from build123d import *

# Parameters (mm, degrees)
BOSS_EXTRUDE1_DEPTH      = 22
BOSS_EXTRUDE1_DEPTH_BACK = 54
SKETCH1_W                = 213
SKETCH1_H                = 136
SKETCH2_W                = 18
SKETCH2_H                = 18
CUT_EXTRUDE1_DEPTH       = 15
CUT_EXTRUDE2_DEPTH       = 12.84
CUT_EXTRUDE3_DEPTH       = 12.84
CUT_EXTRUDE4_DEPTH       = 181.981352631
SKETCH9_R                = 1.905
CUT_EXTRUDE8_DEPTH       = 5
SKETCH11_R               = 4.445
CUT_EXTRUDE10_DEPTH      = 137.921009741


with BuildPart() as part:
    # Sketch1 → Boss-Extrude1 (new, two sides: drawn at the far end of the back side and taken through both)
    with BuildSketch(Plane(origin=(0, 0, 0), x_dir=(1, 0, 0), z_dir=(0, 1, 0)).offset(-BOSS_EXTRUDE1_DEPTH_BACK)):
        Rectangle(SKETCH1_W, SKETCH1_H)
    extrude(amount=BOSS_EXTRUDE1_DEPTH + BOSS_EXTRUDE1_DEPTH_BACK)

    # Sketch2 → Cut-Extrude1 (cut)
    with BuildSketch(Plane(origin=(0, 22, 0), x_dir=(1, 0, 0), z_dir=(0, 1, 0))):
        with Locations((-85.5, 43)):
            Rectangle(SKETCH2_W, SKETCH2_H)
        with Locations((-85.5, -43)):
            Rectangle(SKETCH2_W, SKETCH2_H)
        with Locations((57.5, 43)):
            Rectangle(SKETCH2_W, SKETCH2_H)
        with Locations((57.5, -43)):
            Rectangle(SKETCH2_W, SKETCH2_H)
    extrude(amount=-CUT_EXTRUDE1_DEPTH, mode=Mode.SUBTRACT)

    # Sketch4 → Cut-Extrude2 (cut)
    with BuildSketch(Plane.ZY.offset(76.5)):
        Polygon((34, 7), (52, 7), (52, 11), (48.05, 11), (48.05, 24.194829177), (37.95, 24.194829177), (37.95, 11), (34, 11), align=None)
        Polygon((-34, 7), (-52, 7), (-52, 11), (-48.05, 11), (-48.05, 24.194829177), (-37.95, 24.194829177), (-37.95, 11), (-34, 11), align=None)
    extrude(amount=-CUT_EXTRUDE2_DEPTH, mode=Mode.SUBTRACT)

    # Sketch5 → Cut-Extrude3 (cut)
    with BuildSketch(Plane.ZY.offset(-66.5)):
        Polygon((34, 7), (52, 7), (52, 11), (48.05, 11), (48.05, 24.194829177), (37.95, 24.194829177), (37.95, 11), (34, 11), align=None)
        Polygon((-34, 7), (-52, 7), (-52, 11), (-48.05, 11), (-48.05, 24.194829177), (-37.95, 24.194829177), (-37.95, 11), (-34, 11), align=None)
    extrude(amount=-CUT_EXTRUDE3_DEPTH, mode=Mode.SUBTRACT)

    # Sketch7 → Cut-Extrude4 (cut, through all)
    with BuildSketch(Plane(origin=(0, 0, -68), x_dir=(-1, 0, 0), z_dir=(0, 0, -1))):
        Polygon((106.5, -54), (-106.5, 3.073177988), (-106.5, -54), align=None)
    extrude(amount=-CUT_EXTRUDE4_DEPTH, mode=Mode.SUBTRACT)

    # Sketch9 → Cut-Extrude8 (cut)
    with BuildSketch(Plane(origin=(6.365852752, -23.757685902, 0), x_dir=(0.9659258262890681, 0.2588190451025214, 0), z_dir=(0.2588190451025214, -0.9659258262890681, 0))):
        with Locations((-61.719828935, 0)):
            Circle(SKETCH9_R)
        with Locations((48.538997492, 0)):
            Circle(SKETCH9_R)
    extrude(amount=-CUT_EXTRUDE8_DEPTH, mode=Mode.SUBTRACT)

    # Sketch11 → Cut-Extrude10 (cut, through all)
    with BuildSketch(Plane(origin=(5.071757526, -18.928056771, 0), x_dir=(0.9659258262890681, 0.25881904510252135, 0), z_dir=(0.25881904510252135, -0.9659258262890681, 0))):
        with Locations((-61.719828935, 0)):
            Circle(SKETCH11_R)
        with Locations((48.538997492, 0)):
            Circle(SKETCH11_R)
    extrude(amount=-CUT_EXTRUDE10_DEPTH, mode=Mode.SUBTRACT)


solid = part.part
CAD build for the part. Positions are in the model's coordinates, mm. A direction names the side the tool comes from. Coordinates: 2 decimals unless noted, no trailing zeros. Order: outer loops, then holes, each group sorted by start corner. A loop starts at its lowest first (then second) coordinate and runs counter-clockwise, first axis right, second up.
Item 1: Band-saw the part on B-B on y = -45. List the corners of the cut face in (x, z).
Check sheet entries:
outline: (-106.5, -68) - (-72.91, -68) - (-72.91, 68) - (-106.5, 68) - close
Item 2: Pin check, flat tips, straight feed: pin 1 Ø2 at (x, z) = (71, -50) entering from -Y; pin 2 Ø1.2 at (x, z) = (74.5, 35.5) entering from -Y; pin 3 Ø1.5 at (x, z) = (-33.5, -46) entering from -Y. Stop position of each tip, or through.
Check sheet entries:
pin 1: stops at y = -6.71
pin 2: stops at y = -5.66
pin 3: stops at y = -34.64
Item 3: Two-plate mould, pull along Z, no slides. Class faces 4 (the face through (-25, -8, 68)), 5 (the face through (-106.5, -17, 1)), 6 (the face through (-79, 7, -43)): +Z half, -Z half, draft (parallel to the pull), parting line (faces both ways), or undercut.
Check sheet entries:
face 4: +Z half
face 5: draft
face 6: undercut
Item 4: Band-saw the part on C-C on z = 20. List the corners of the cut face in (x, y).
Check sheet entries:
outline: (-106.5, -54) - (106.5, 3.07) - (106.5, 22) - (-106.5, 22) - close
Item 5: 3-axis set-ups, long thin cutter, end or side, ignore diameter. For faces 1 (the face through (-25, -8, -68)), 2 (the face through (-83, 13, 34)), 3 (the face through (-70, 17, -37.95)): which of +Z, -Z, +X, -X, +Y, -Y reach the whole face in a straight line?
Check sheet entries:
face 1: -Z, +X, -X, +Y, -Y
face 2: none
face 3: +Y
Item 6: Band-saw the part on D-D on y = 14. Give the number of separate pieces and of enclosed holes in the cut face, plus the area to 3 significant figures.
Check sheet entries:
separate pieces: 1
enclosed holes: 6
area: 27,000 mm2
Item 7: Band-saw the part on A-A on x = 76.5. List the corners of the cut face in (y, z), plus the area to 3 significant figures.
Check sheet entries:
outline: (-4.97, -68) - (22, -68) - (22, -48.05) - (11, -48.05) - (11, -52) - (7, -52) - (7, -34) - (11, -34) - (11, -37.95) - (22, -37.95) - (22, 37.95) - (11, 37.95) - (11, 34) - (7, 34) - (7, 52) - (11, 52) - (11, 48.05) - (22, 48.05) - (22, 68) - (-4.97, 68) - close
area: 3,300 mm2
Item 8: Drill centre lines: L1, parallel to X at y = 16, z = -42.5; L2, parallel to Y at x = -31, z = 22; L3, parallel to Y at x = 71.5, z = 50. Where is each one in solid material? Low to high.
Check sheet entries:
L1: x = -106.5 to -94.5, -63.66 to 48.5, 79.34 to 106.5
L2: y = -33.77 to 22
L3: y = -6.31 to 7, 11 to 22
